The model under review builds one solid part; all positions refer to its coordinate system, in mm. Face numbers are marked on the shaded views. A direction names the side the tool comes from. Coordinates: 2 decimals unless noted, no trailing zeros. Order: outer loops, then holes, each group sorted by start corner. A loop starts at its lowest first (then second) coordinate and runs counter-clockwise, first axis right, second up. Notation, with made-up numbers: M 63,0.5 L 105,0.5 A20 cw 105,33.5 Z; hole C 17,62.5 d5. An arc over 180 degrees is marked long. Answer in a Markdown table with one row per item.
from build123d import *

# Parameters (mm, degrees)
SKETCH119_W             = 2
SKETCH119_H             = 6
POCKET017_DEPTH         = 2
CHAMFER006_SIZE         = 0.35
CHAMFER007_SIZE         = 0.75
BODY020_PLACEMENT_ANGLE = 90
BODY019_PLACEMENT_ANGLE = 90


with BuildPart() as part:
    # Sketch119 → Revolution002 (revolve)
    with BuildSketch(Plane.XZ):
        with Locations((-1, 3)):
            Rectangle(SKETCH119_W, SKETCH119_H)
    revolve(axis=Axis((0, 0, 0), (0, 0, 1)))

    # Sketch124 (on Face3 of Revolution002) → Pocket017 (cut)
    with BuildSketch(Plane(origin=(0, 0, 6), x_dir=(-1, 0, 0), z_dir=(0, 0, 1))):
        Polygon((-0.625, -1.0825317547), (0.625, -1.0825317547), (1.25, 0), (0.625, 1.0825317547), (-0.625, 1.0825317547), (-1.25, 0), align=None)
    extrude(amount=-POCKET017_DEPTH, mode=Mode.SUBTRACT)

    # Chamfer006
    chamfer006_edges = [part.edges().sort_by_distance(p)[0] for p in [
        (2, 0, 6),
    ]]
    chamfer(chamfer006_edges, length=CHAMFER006_SIZE)

    # Chamfer007
    chamfer007_edges = [part.edges().sort_by_distance(p)[0] for p in [
        (2, 0, 0),
    ]]
    chamfer(chamfer007_edges, length=CHAMFER007_SIZE)


with BuildPart() as part_1:
    # Body020 placement: moved
    add(part.part.moved(Location((0, -3, 4))).rotate(Axis((0, -3, 4), (1, 0, 0)), BODY020_PLACEMENT_ANGLE))


with BuildPart() as part_2:
    # Clone002 placement: moved
    add(part_1.part.moved(Location((0, -1, 0))))


with BuildPart() as part_3:
    # Body019 placement: moved
    add(part_2.part.moved(Location((-1, 0, 0))).rotate(Axis((-1, 0, 0), (0, 0, 1)), BODY019_PLACEMENT_ANGLE))


solid = part_3.part
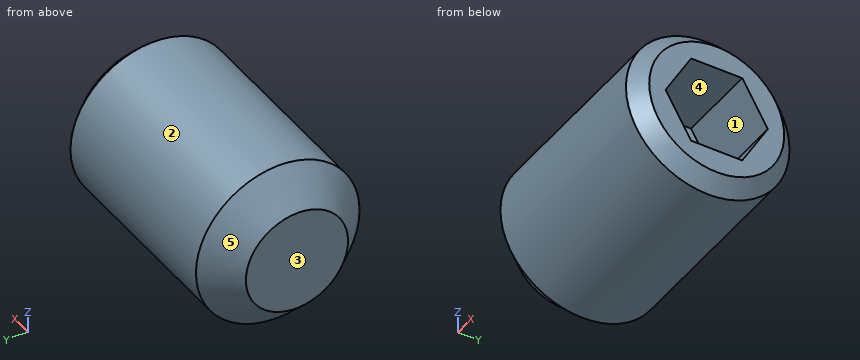
(1) Take a section at D-D (x = 3.5). Write out the cut boundary in (y, z), then the cut area to 3 significant figures.
Report:
| item | result |
|---|---|
| outline | C 0,4 d3.5 |
| area | 9.62 mm^2 |
(2) Machinability: for the marked faces 4 and 5, which of the approach directions +Z, -Z, +X, -X, +Y, -Y give a long, thin tool a straight path to every point of the face, cutting with its end or side? Answer none if there is none.
Report:
| item | result |
|---|---|
| face 4 | +X |
| face 5 | -X |
(3) Take a section at C-C (x = 6.05). Write out the cut boundary in (y, z).
Report:
| item | result |
|---|---|
| outline | C 0,4 d4 |
(4) Take a section at A-A (x = 7.6). Write out the cut boundary in (y, z) (3 decimals).
Report:
| item | result |
|---|---|
| outline | C 0,4 d4; hole M -1.25,4 L -0.625,2.917 L 0.625,2.917 L 1.25,4 L 0.625,5.083 L -0.625,5.083 Z |
(5) Insertion check: P1, Ø1, axis at x = 8.5, z = 5.5, coming from the +Y side; P2, Ø1, axis at x = 3.5, y = 1, coming from the +Z side; P3, Ø1.5, axis at x = 5.5, z = 2.5, coming from the +Y side. Each pin has a flat end and moves straight along its axis. Give the tip position at first contact, or say it passes through.
Report:
| item | result |
|---|---|
| P1 | y = 1.73 |
| P2 | z = 5.92 |
| P3 | y = 1.85 |
(6) To check wall thickness, follow line 1 (Z direction, x = 8.6, y = -0.05); line 2 (X direction, y = 0.25, z = 4.8); line 3 (Z direction, x = 7.65, y = 1.15). State the ranges of each line that lie inside material, in increasing order. Write a range as [from, to].
Report:
| item | result |
|---|---|
| line 1 | [2, 2.92], [5.08, 6] |
| line 2 | [3, 7] |
| line 3 | [2.36, 3.83], [4.17, 5.64] |
(7) The part is to be moulded in two halves that separate along Y. For the marked faces 1, 2 and 3, say which applies: +Y half, -Y half, draft (parallel to the pull), parting line (faces both ways), or undercut.
Report:
| item | result |
|---|---|
| face 1 | undercut |
| face 2 | parting line |
| face 3 | draft |
(8) Take a section at B-B (y = 0). Write out the cut boundary in (x, z), then the cut area to 3 significant figures.
Report:
| item | result |
|---|---|
| outline | M 3,2.75 L 3.75,2 L 8.65,2 L 9,2.35 L 9,2.92 L 7,2.92 L 7,5.08 L 9,5.08 L 9,5.65 L 8.65,6 L 3.75,6 L 3,5.25 Z |
| area | 19.0 mm^2 |
